Could you check a few things on this model? Use its own coordinates, in mm. Round coordinates to 2 decimals unless told otherwise and drop trailing zeros. Write each loop counter-clockwise with the first axis right and the second up, starting at its lowest first coordinate (ties: lowest second). Pieces come first, ordered by that corner, then holes.
Autodesk Inventor part; units mm, degrees
ref_plane "YZ Plane" through (0, 0, 0) normal (1, 0, 0) x (0, 1, 0)
ref_plane "XZ Plane" through (0, 0, 0) normal (0, 1, 0) x (-1, 0, 0)
ref_plane "XY Plane" through (0, 0, 0) normal (0, 0, 1) x (1, 0, 0)
sketch "Sketch1" plane through (0, 0, 0) normal (0, 1, 0) x (-1, 0, 0)
  circle A0 centre (0, 0) radius 2
  line L0 (-3.4641, -6) -> (3.4641, -6)
  line L1 (3.4641, -6) -> (6.9282, 0)
  line L2 (6.9282, 0) -> (3.4641, 6)
  line L3 (3.4641, 6) -> (-3.4641, 6)
  line L4 (-3.4641, 6) -> (-6.9282, 0)
  line L5 (-6.9282, 0) -> (-3.4641, -6)
  line L6 (0, 6) -> (0, -6) construction
  line L7 (-5.1962, 3) -> (5.1962, -3) construction
  line L8 (-5.1962, -3) -> (5.1962, 3) construction
  point P0 (0, 0)
  dimension "d0" = 4
  dimension "d1" = 12
extrude "Extrusion1" add sketch "Sketch1" along normal blind 4
offset faces "Size1" outward -0.18 faces at (-1.9935, 2.6667, -0.1609)
properties part number "Front_Wheel_Support_Test"
Q1. We'd pull the mould along Z, two halves only. Please class faces 1 (the flat face through (5.172, 1.972, 3.042)), 2 (the cylindrical face through (0.47, 1.97, 2.13)), 3 (the flat face through (-3, 4, 0)): pulls with the +Z half, pulls with the -Z half, needs draft (parallel to the pull), parting line crosses it, or undercut.
Q2. If I drill on L1, parallel to Z at x = 0, y = 1.6; L2, parallel to X at y = 0.85, z = -1.5; L3, parallel to X at y = 1.3, z = -0.5, over which ranges is the centre line in solid material (lowest first)?
Q3. Imagine slicing it at A-A, the plane x = 0. Write out the boundary of the cut face in (y, z), then the cut area to 3 significant figures.
Q4. Imagine slicing it at B-B, the plane y = 1.7. Write out the boundary of the cut face in (x, z).
Q5. I'm going to push flat-ended pins straight in: pin 1 Ø2 at (y, z) = (1, 4) entering from +X; pin 2 Ø4 at (x, z) = (0.5, 0) entering from -Y; pin 3 Ø1 at (x, y) = (-5.5, 3.5) entering from +Z; pin 4 Ø2 at (y, z) = (2.5, -3) entering from +X. Where does each tip first touch, or does it pass through?
Q6. Imagine slicing it at D-D, the plane x = 1.5. Write out the boundary of the cut face in (y, z).
Q7. Imagine slicing it at C-C, the plane z = 3. Write out the boundary of the cut face in (x, y), then the cut area to 3 significant figures.
Results found:
1. face 1: pulls with the +Z half
1. face 2: undercut
1. face 3: needs draft
2. L1: z = -6 to -2.18, 2.18 to 6
2. L2: x = -6.06 to -1.58, 1.58 to 6.06
2. L3: x = -6.64 to -2.12, 2.12 to 6.64
3. outline: (0, -6) - (4, -6) - (4, -2.18) - (0, -2.18) - close; (0, 2.18) - (4, 2.18) - (4, 6) - (0, 6) - close
3. area: 30.6 mm2
4. outline: (-6.93, 0) - (-3.46, -6) - (3.46, -6) - (6.93, 0) - (3.46, 6) - (-3.46, 6) - close; hole circle Ø4.36 at (0, 0)
5. pin 1: stops at x = 5.2
5. pin 2: stops at y = 0
5. pin 3: stops at z = 3.34
5. pin 4: stops at x = 5.77
6. outline: (0, -6) - (4, -6) - (4, -1.58) - (0, -1.58) - close; (0, 1.58) - (4, 1.58) - (4, 6) - (0, 6) - close
7. outline: (-5.2, 0) - (5.2, 0) - (5.2, 4) - (-5.2, 4) - close
7. area: 41.6 mm2
